Read the model definition and answer for the solid it produces. Units are mm, in the model's axes. A direction names the side the tool comes from. Round coordinates to 2 decimals unless told otherwise and drop trailing zeros. Write each loop counter-clockwise with the first axis right and the second up, starting at its lowest first coordinate (ties: lowest second). Pieces come first, ordered by that corner, then holes. Notation, with made-up numbers: (-11.5, 83) - (2.5, 83) arc R17 ccw to (2.5, 87) - close; hole circle Ø7 at (64.25, 73). An arc over 180 degrees is marked (long way). One line per item, written item: value. Start each with the question number.
(1) The mould has two halves that part along X. Classify faces 3 (the face through (165.1, 5, -138)), 4 (the face through (81, 0, -142)), 5 (the face through (9.5, 4.699, -31.8)): +X half, -X half, draft (parallel to the pull), parting line (faces both ways), or undercut.
(2) A cutting plane is placed at B-B, the plane z = -266.7. Determine the outline of the cut face in (x, y) (3 decimals).
(3) Flat-ended cylindrical pins translate along their axes: pin 1 Ø5 at (x, z) = (6.35, -31.75) entering from -Y; pin 2 Ø7 at (x, z) = (20.828, -49.53) entering from +Y. Find the tip coordinate at first contact, or state that the pin passes through.
(4) For faces 1 (the face through (157.72, 7.15, -243)), 2 (the face through (156.157, 2.317, -30.675)), determine the directions among +Z, -Z, +X, -X, +Y, -Y from which every point of the face is accessible in a straight line to the end or side of a thin tool.
(5) A cutting plane is placed at A-A, the plane x = 6.35. Determine the outline of the cut face in (y, z) (1 decimal).
(6) Find the intervals of material crossed by L1, parallel to X at y = 1.4, z = -31.75; L2, parallel to X at y = 8, z = -49; L3, parallel to Z at x = 158.75, y = 6.8, in increasing order.
from build123d import *

# Parameters (mm, degrees)
SKETCH1_W                                       = 165.1
SKETCH1_H                                       = 279.4
BOSS_EXTRUDE1_DEPTH                             = 9.525
F_1_4_CLEARANCE_HOLE1_D                         = 7.14248
CBORE_FOR_10_SOCKET_HEAD_CAP_SCREW1_D           = 5.6134
CBORE_FOR_10_SOCKET_HEAD_CAP_SCREW1_CBORE_D     = 9.525
CBORE_FOR_10_SOCKET_HEAD_CAP_SCREW1_CBORE_DEPTH = 4.826
CBORE_FOR_6_SOCKET_HEAD_CAP_SCREW1_D            = 4.3053
CBORE_FOR_6_SOCKET_HEAD_CAP_SCREW1_CBORE_D      = 7.14502
CBORE_FOR_6_SOCKET_HEAD_CAP_SCREW1_CBORE_DEPTH  = 3.5052


with BuildPart() as part:
    # Sketch1 → Boss-Extrude1 (new body)
    with BuildSketch(Plane(origin=(0, 0, 0), x_dir=(1, 0, 0), z_dir=(0, 1, 0))):
        with Locations((82.55, 139.7)):
            Rectangle(SKETCH1_W, SKETCH1_H)
    extrude(amount=BOSS_EXTRUDE1_DEPTH)

    # 1/4 Clearance Hole1 (through all)
    with Locations(Plane(origin=(0, 9.525, 0), x_dir=(1, 0, 0), z_dir=(0, 1, 0))):
        with Locations((152.4, 12.7), (12.7, 12.7), (12.7, 266.7), (152.4, 266.7)):
            Hole(F_1_4_CLEARANCE_HOLE1_D / 2)

    # CBORE for #10 Socket Head Cap Screw1 (through all)
    with Locations(Plane(origin=(0, 9.525, 0), x_dir=(1, 0, 0), z_dir=(0, 1, 0))):
        with Locations((6.35, 247.65), (6.35, 31.75), (158.75, 31.75), (158.75, 247.65)):
            CounterBoreHole(CBORE_FOR_10_SOCKET_HEAD_CAP_SCREW1_D / 2, CBORE_FOR_10_SOCKET_HEAD_CAP_SCREW1_CBORE_D / 2, CBORE_FOR_10_SOCKET_HEAD_CAP_SCREW1_CBORE_DEPTH)

    # CBORE for #6 Socket Head Cap Screw1 (through all)
    with Locations(Plane(origin=(0, 9.525, 0), x_dir=(1, 0, 0), z_dir=(0, 1, 0))):
        with Locations((144.272, 229.87), (144.272, 49.53), (20.828, 49.53), (20.828, 208.28)):
            CounterBoreHole(CBORE_FOR_6_SOCKET_HEAD_CAP_SCREW1_D / 2, CBORE_FOR_6_SOCKET_HEAD_CAP_SCREW1_CBORE_D / 2, CBORE_FOR_6_SOCKET_HEAD_CAP_SCREW1_CBORE_DEPTH)


solid = part.part
Here are the results:
1. face 3: +X half
1. face 4: draft
1. face 5: undercut
2. outline: (0, 0) - (9.129, 0) - (9.129, 9.525) - (0, 9.525) - close; (16.271, 0) - (148.829, 0) - (148.829, 9.525) - (16.271, 9.525) - close; (155.971, 0) - (165.1, 0) - (165.1, 9.525) - (155.971, 9.525) - close
3. pin 1: through
3. pin 2: y = 6.02
4. face 1: +Y
4. face 2: +Y, -Y
5. outline: (0, -279.4) - (9.5, -279.4) - (9.5, -252.4) - (4.7, -252.4) - (4.7, -250.5) - (0, -250.5) - close; (0, -244.8) - (4.7, -244.8) - (4.7, -242.9) - (9.5, -242.9) - (9.5, -36.5) - (4.7, -36.5) - (4.7, -34.6) - (0, -34.6) - close; (0, -28.9) - (4.7, -28.9) - (4.7, -27) - (9.5, -27) - (9.5, 0) - (0, 0) - close
6. L1: 0 to 3.54, 9.16 to 155.94, 161.56 to 165.1
6. L2: 0 to 17.3, 24.36 to 140.74, 147.8 to 165.1
6. L3: -279.4 to -252.41, -242.89 to -36.51, -26.99 to 0
